Work out the finished part from the listing and answer in its coordinate system (mm). Round coordinates to 2 decimals unless told otherwise and drop trailing zeros. Write each loop counter-clockwise with the first axis right and the second up, starting at its lowest first coordinate (ties: lowest second). Pieces come first, ordered by that corner, then holes. Notation, with made-up numbers: M 27,74 L 81,74 A24 ccw 81,111 Z; hole C 41,-3 d4. An arc over 180 degrees is marked long. Answer in a Markdown table with one row per item.
```python
from build123d import *

# Parameters (mm, degrees)
SKETCH1_W                  = 25.4
SKETCH1_H                  = 25.4
SKETCH1_W_2                = 22.098
SKETCH1_H_2                = 22.098
BOSS_EXTRUDE1_DEPTH        = 508
FILLET1_R                  = 1.27
F_1_0_228_DIAMETER_HOLE2_D = 5.7912
F_1_0_228_DIAMETER_HOLE3_D = 5.7912


with BuildPart() as part:
    # Sketch1 → Boss-Extrude1 (new body)
    with BuildSketch(Plane(origin=(0, 0, 0), x_dir=(1, 0, 0), z_dir=(0, 1, 0))):
        Rectangle(SKETCH1_W, SKETCH1_H)
        Rectangle(SKETCH1_W_2, SKETCH1_H_2, mode=Mode.SUBTRACT)
    extrude(amount=BOSS_EXTRUDE1_DEPTH)

    # Fillet1
    fillet1_edges = [part.edges().sort_by_distance(p)[0] for p in [
        (-11.049, 254, 11.049),
        (11.049, 254, 11.049),
        (11.049, 254, -11.049),
        (-11.049, 254, -11.049),
        (12.7, 254, 12.7),
        (-12.7, 254, 12.7),
        (-12.7, 254, -12.7),
        (12.7, 254, -12.7),
    ]]
    fillet(fillet1_edges, radius=FILLET1_R)

    # #1 (0.228) Diameter Hole2 (through all)
    with Locations(Plane.ZY.offset(12.7)):
        with Locations((0, 463.55), (0, 44.45), (0, 254)):
            Hole(F_1_0_228_DIAMETER_HOLE2_D / 2)

    # #1 (0.228) Diameter Hole3 (through all)
    with Locations(Plane(origin=(0, 0, -12.7), x_dir=(-1, 0, 0), z_dir=(0, 0, -1))):
        with Locations((0, 420.6875), (0, 87.3125)):
            Hole(F_1_0_228_DIAMETER_HOLE3_D / 2)


solid = part.part
```
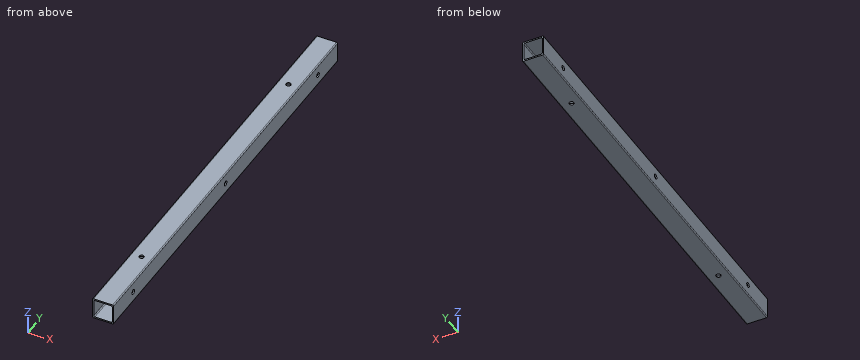
1. Consider line 1 along Y through (x, z) = (11.75, 0); line 2 along Y through (x, z) = (0, 12.3); line 3 along Z through (x, y) = (8, 483). Determine where each line is inside the solid, lowest interval first. Write a range as from..to.
Calculated:
| item | result |
|---|---|
| line 1 | y = 0..41.55, 47.35..251.1, 256.9..460.65, 466.45..508 |
| line 2 | y = 0..84.42, 90.21..417.79, 423.58..508 |
| line 3 | z = -12.7..-11.05, 11.05..12.7 |
2. Given pin 1 (7.5 mm diameter, centred on x = 0, y = 420.69, fed in from +Z); pin 2 (4.5 mm diameter, centred on y = 254, z = 0, fed in from -X), each flat-ended and moving along its own axis, determine where each tip first touches the part or whether it passes through.
Calculated:
| item | result |
|---|---|
| pin 1 | stops at z = 12.7 |
| pin 2 | passes through |
3. The part is cut by section A-A (y = 438.5). Determine the outline of the cut face in (x, z), plus the area to 3 significant figures.
Calculated:
| item | result |
|---|---|
| outline | M -12.7,-11.43 A1.27 ccw -11.43,-12.7 L 11.43,-12.7 A1.27 ccw 12.7,-11.43 L 12.7,11.43 A1.27 ccw 11.43,12.7 L -11.43,12.7 A1.27 ccw -12.7,11.43 Z; hole M -11.05,-9.78 A1.27 ccw -9.78,-11.05 L 9.78,-11.05 A1.27 ccw 11.05,-9.78 L 11.05,9.78 A1.27 ccw 9.78,11.05 L -9.78,11.05 A1.27 ccw -11.05,9.78 Z |
| area | 157 mm² |
